Here's the drawing with two shaded views (mm, measured from the low corner). I have some questions. A direction names the side the tool comes from. Round coordinates to 2 decimals unless told otherwise and drop trailing zeros. Loops run counter-clockwise (first coordinate to the right, second up) from the corner with the lowest first, then second, coordinate; pieces in that order, holes last. Notation, with made-up numbers: (28.5, 67.5) - (60.5, 67.5) arc R17 cw to (60.5, 81.5) - close; hole circle Ø11 at (81, 75.25). An arc over 180 degrees is marked (long way). Use one line per item in the form item = value.
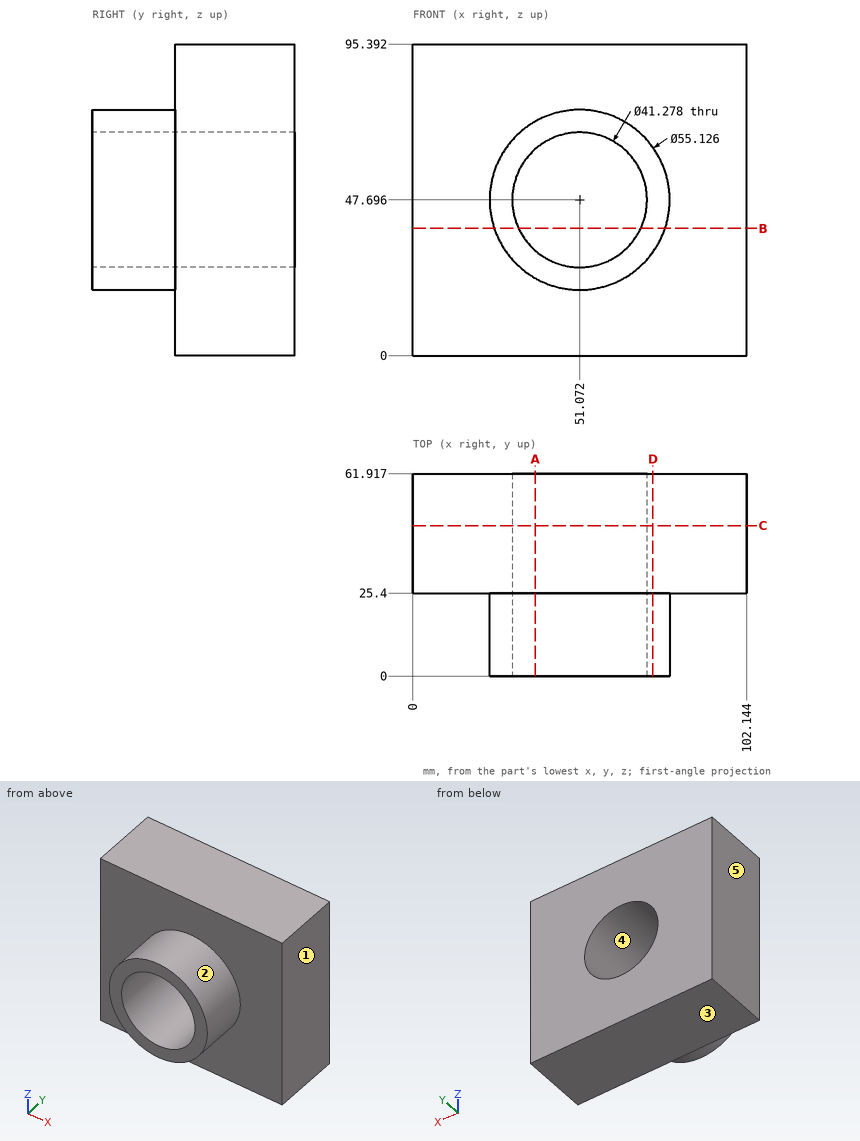
1. If we section it at B-B, the plane z = 39: Write out the boundary of the cut face in (x, y) (1 decimal).
Solution:
outline = (0, 25.4) - (24.9, 25.4) - (24.9, 0) - (32.4, 0) - (32.4, 61.9) - (0, 61.9) - close; (69.8, 0) - (77.2, 0) - (77.2, 25.4) - (102.1, 25.4) - (102.1, 61.9) - (69.8, 61.9) - close
2. We'd pull the mould along X, two halves only. Please class the marked faces 3, 4 and 5: +X half, -X half, draft (parallel to the pull), parting line (faces both ways), or undercut.
Solution:
face_3 = draft
face_4 = undercut
face_5 = -X half
3. Please list where these lines run through material, in increasing order: line 1 along Y through (x, z) = (98, 91.5); line 2 along Z through (x, y) = (50, 38.5) (1 decimal); line 3 along X through (y, z) = (46, 29.5) (1 decimal).
Solution:
line_1 = 25.4 to 61.92
line_2 = 0 to 27.1, 68.3 to 95.4
line_3 = 0 to 41.3, 60.8 to 102.1
4. If we section it at C-C, the plane y = 46: Write out the boundary of the cut face in (x, z) (1 decimal), plus the area to 3 significant figures.
Solution:
outline = (0, 0) - (102.1, 0) - (102.1, 95.4) - (0, 95.4) - close; hole circle Ø41.3 at (51.1, 47.7)
area = 8,410 mm^2
5. If we section it at A-A, the plane x = 37.5: Write out the boundary of the cut face in (y, z) (1 decimal), plus the area to 3 significant figures.
Solution:
outline = (0, 23.7) - (25.4, 23.7) - (25.4, 0) - (61.9, 0) - (61.9, 32.1) - (0, 32.1) - close; (0, 63.2) - (61.9, 63.2) - (61.9, 95.4) - (25.4, 95.4) - (25.4, 71.7) - (0, 71.7) - close
area = 2,780 mm^2
6. For P1, Ø6, axis at y = 18.5, z = 75.5, coming from the -X side, with a flat end and sliding along its axis, tell me the tip position at first contact or that it passes through.
Solution:
P1 = 39.05
7. If we section it at D-D, the plane x = 73.5: Write out the boundary of the cut face in (y, z), plus the area to 3 significant figures.
Solution:
outline = (0, 31.67) - (25.4, 31.67) - (25.4, 0) - (61.92, 0) - (61.92, 95.39) - (25.4, 95.39) - (25.4, 63.72) - (0, 63.72) - close
area = 4,300 mm^2
8. On a 3-axis mill with a long thin cutter (end or side, diameter ignored), from which of +Z, -Z, +X, -X, +Y, -Y can I reach the whole of each face in a straight line? I mean the marked faces 1 and 2. Say none if no direction works.
Solution:
face_1 = +Z, -Z, +X, +Y, -Y
face_2 = -Y
